Geometry check sheet. Reference: the model listing, model coordinates, mm. Face numbers are marked on the shaded views. A direction names the side the tool comes from. Round coordinates to 2 decimals unless told otherwise and drop trailing zeros. Loops run counter-clockwise (first coordinate to the right, second up) from the corner with the lowest first, then second, coordinate; pieces in that order, holes last.
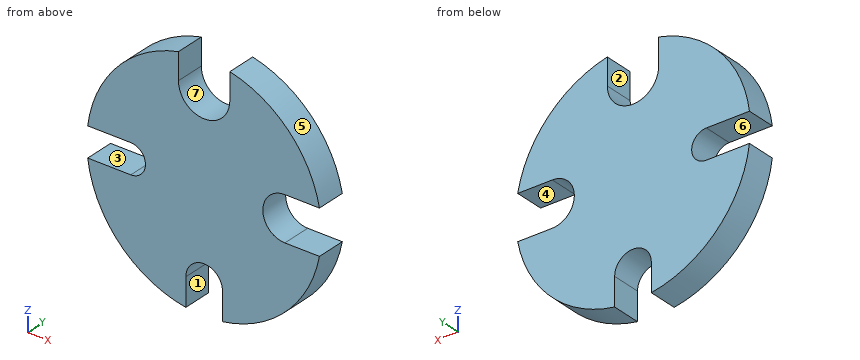
```python
from build123d import *

# Parameters (mm, degrees)
BOSS_EXTRUDE1_DEPTH = 25.4


with BuildPart() as part:
    # Sketch1 → Boss-Extrude1 (new body)
    with BuildSketch(Plane(origin=(0, 0, 0), x_dir=(1, 0, 0), z_dir=(0, 1, 0))):
        with BuildLine():
            ThreePointArc((-100.803124952, -12.7), (-75.179251769, -68.342081498), (-22.225, -99.139343225))
            Line((-22.225, -99.139343225), (-22.225, -76.2))
            ThreePointArc((-22.225, -76.2), (0, -53.975), (22.225, -76.2))
            Line((22.225, -76.2), (22.225, -99.139343225))
            ThreePointArc((22.225, -99.139343225), (72.97933927, -70.686462917), (99.798083649, -19.05))
            Line((99.798083649, -19.05), (69.85, -19.05))
            ThreePointArc((69.85, -19.05), (50.8, 0), (69.85, 19.05))
            Line((69.85, 19.05), (99.798083649, 19.05))
            ThreePointArc((99.798083649, 19.05), (70.693518214, 72.972504977), (15.875, 100.352101996))
            Line((15.875, 100.352101996), (15.875, 76.2))
            ThreePointArc((15.875, 76.2), (0, 60.325), (-15.875, 76.2))
            Line((-15.875, 76.2), (-15.875, 100.352101996))
            ThreePointArc((-15.875, 100.352101996), (-72.966903159, 70.699300162), (-100.803124952, 12.7))
            Line((-100.803124952, 12.7), (-63.5, 12.7))
            ThreePointArc((-63.5, 12.7), (-50.8, 0), (-63.5, -12.7))
            Line((-63.5, -12.7), (-100.803124952, -12.7))
        make_face()
    extrude(amount=BOSS_EXTRUDE1_DEPTH)


solid = part.part
```
1) Sectioned sample at A-A, the plane z = 69. Record the cut outline in (x, y).
Report:
outline: (-74.58, 0) - (-21.03, 0) - (-21.03, 25.4) - (-74.58, 25.4) - close; (21.03, 0) - (74.58, 0) - (74.58, 25.4) - (21.03, 25.4) - close
2) Mould release check, pull along X, two halves, no side actions. Record for the marked faces 5, 6 and 7: +X half, -X half, draft (parallel to the pull), parting line (faces both ways), or undercut.
Report:
face 5: +X half
face 6: draft
face 7: undercut
3) Sectioned sample at B-B, the plane x = -87. Record the cut outline in (y, z).
Report:
outline: (0, -52.47) - (25.4, -52.47) - (25.4, -12.7) - (0, -12.7) - close; (0, 12.7) - (25.4, 12.7) - (25.4, 52.47) - (0, 52.47) - close
4) Scan lines: line 1 along X through (y, z) = (8.5, -84) (3 decimals); line 2 along X through (y, z) = (17.75, 77.5) (3 decimals); line 3 along Z through (x, y) = (-57.5, 11.5). Record each from-to range of solid material in increasing order.
Report:
line 1: x = -57.154 to -15.875, 15.875 to 57.154
line 2: x = -65.699 to -22.225, 22.225 to 65.699
line 3: z = -83.76 to -11.19, 11.19 to 83.76
5) Sectioned sample at D-D, the plane z = 0. Record the cut outline in (x, y), then the cut area to 3 significant figures.
Report:
outline: (-50.8, 0) - (50.8, 0) - (50.8, 25.4) - (-50.8, 25.4) - close
area: 2,580 mm2
6) Gauge pin test, flat ends, axial feed: pin 1 (1.5 mm diameter, centred on y = 4.5, z = 43, fed in from -X); pin 2 (2 mm diameter, centred on x = -33.5, y = 5.5, fed in from -Z); pin 3 (4 mm diameter, centred on x = 40.5, y = 16, fed in from -Z). Record the tip position at first contact, or that the pin passes through.
Report:
pin 1: stops at x = -92.4
pin 2: stops at z = -96.26
pin 3: stops at z = -94.02
7) Sectioned sample at C-C, the plane y = 19.25. Record the cut outline in (x, z) (3 decimals), then the cut area to 3 significant figures.
Report:
outline: (-100.803, -12.7) arc R101.6 ccw to (-15.875, -100.352) - (-15.875, -76.2) arc R15.875 cw to (15.875, -76.2) - (15.875, -100.352) arc R101.6 ccw to (99.798, -19.05) - (69.85, -19.05) arc R19.05 cw to (69.85, 19.05) - (99.798, 19.05) arc R101.6 ccw to (22.225, 99.139) - (22.225, 76.2) arc R22.225 cw to (-22.225, 76.2) - (-22.225, 99.139) arc R101.6 ccw to (-100.803, 12.7) - (-63.5, 12.7) arc R12.7 cw to (-63.5, -12.7) - close
area: 26,400 mm2
8) Access from +Z, -Z, +X, -X, +Y, -Y to the whole of each face (thin tool, end or side, straight path). Record for the marked faces 1, 2, 3 and 4.
Report:
face 1: -Z, +Y, -Y
face 2: +Z, +Y, -Y
face 3: -X, +Y, -Y
face 4: +X, +Y, -Y
